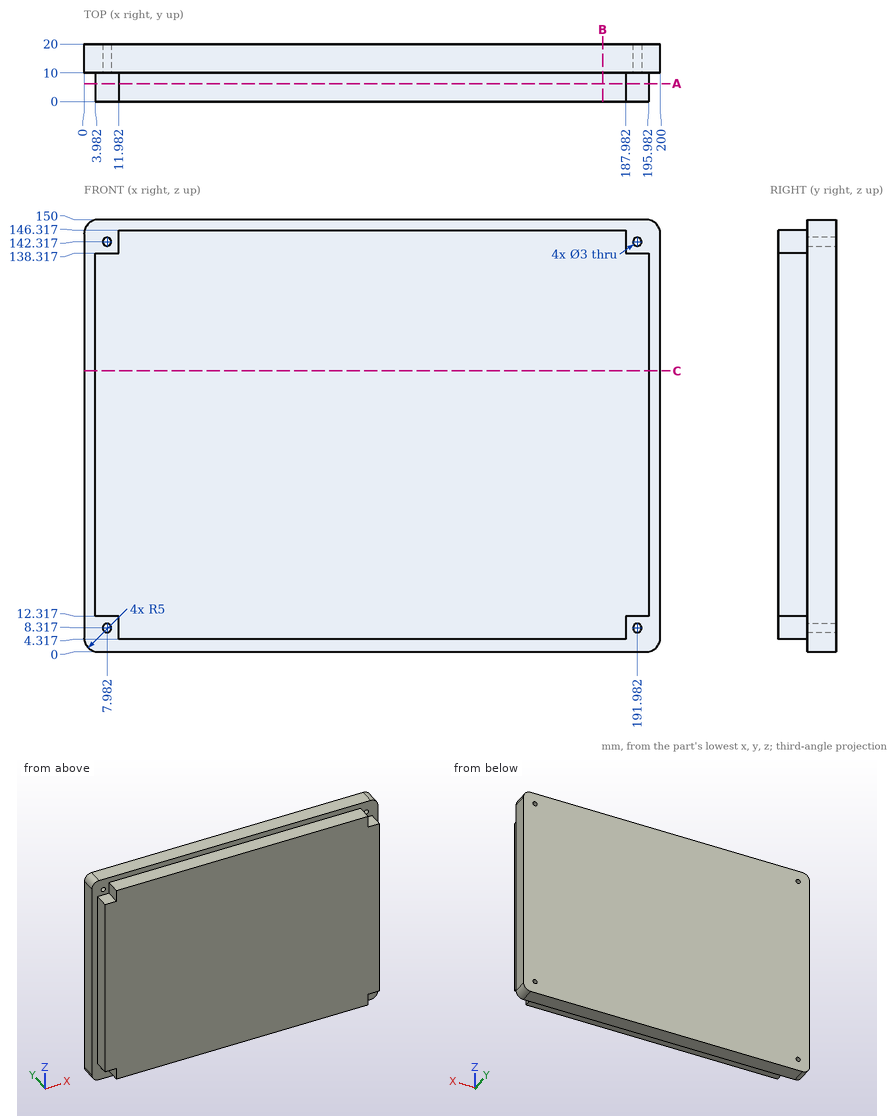
Geometry: see drawing. Coordinates: mm, zero at the bounding-box minimum. Give positions to 0.01 mm unless a question says otherwise; leave off trailing zeros. Loops run counter-clockwise (first coordinate to the right, second up) from the corner with the lowest first, then second, coordinate; pieces in that order, holes last. Notation, with made-up numbers: (-18.5, -31) -> (-10.5, -31) arc R21 cw to (-10.5, -3) -> close; hole circle Ø3 at (81, 70). An arc over 180 degrees is marked (long way). Answer as a JSON object with one key per item and string values. Group by question number.
Item 1: Cut plane A-A, the plane y = 6.25. Return the cut outline in (x, z).
Item 2: Pin query (flat end, axial travel): P1, Ø3, axis at y = 2.5, z = 85, coming from the +X side; P2, Ø5, axis at x = 135.5, y = 4.5, coming from the +Z side; P3, Ø3.5, axis at x = 7.98, z = 142.32, coming from the +Y side; P4, Ø3.5, axis at x = 7.98, z = 8.32, coming from the -Y side. Return the tip coordinate at first contact, or that it passes through.
Item 3: Cut plane B-B, the plane x = 180. Return the cut outline in (y, z), and give its area (3 significant figures).
Item 4: Cut plane C-C, the plane z = 97.5. Return the cut outline in (x, y).
Item 5: Line query: probe 1 along Z at (x, y) = (22, 6.5); probe 2 along X at (y, z) = (6.5, 67); probe 3 along Z at (x, y) = (191, 4). Output: solid intervals per line, ascending.
Checks:
{
 "1": {"outline": "(3.98, 12.32) -> (11.98, 12.32) -> (11.98, 4.32) -> (187.98, 4.32) -> (187.98, 12.32) -> (195.98, 12.32) -> (195.98, 138.32) -> (187.98, 138.32) -> (187.98, 146.32) -> (11.98, 146.32) -> (11.98, 138.32) -> (3.98, 138.32) -> close"},
 "2": {"P1": "stops at x = 195.98", "P2": "stops at z = 146.32", "P3": "stops at y = 20", "P4": "stops at y = 10"},
 "3": {"outline": "(0, 4.32) -> (10, 4.32) -> (10, 0) -> (20, 0) -> (20, 150) -> (10, 150) -> (10, 146.32) -> (0, 146.32) -> close", "area": "2,920 mm²"},
 "4": {"outline": "(0, 10) -> (3.98, 10) -> (3.98, 0) -> (195.98, 0) -> (195.98, 10) -> (200, 10) -> (200, 20) -> (0, 20) -> close"},
 "5": {"probe 1": "z = 4.32 to 146.32", "probe 2": "x = 3.98 to 195.98", "probe 3": "z = 12.32 to 138.32"}
}
